```python
from build123d import *

# Parameters (mm, degrees)
SKETCH2_W           = 50
SKETCH2_H           = 60
BOSS_EXTRUDE1_DEPTH = 25
SHELL1_T            = -3
SKETCH3_R           = 11
BOSS_EXTRUDE2_DEPTH = 3
SKETCH4_R           = 4.5
SKETCH4_R_2         = 1
CUT_EXTRUDE1_DEPTH  = 6
CUT_EXTRUDE2_REACH  = 83.24
CUT_EXTRUDE4_REACH  = 83.24
SKETCH7_W           = 4.336684694
SKETCH7_H           = 5
SKETCH7_W_2         = 5
SKETCH7_H_2         = 4.336684694
BOSS_EXTRUDE3_DEPTH = 44
BOSS_EXTRUDE4_REACH = 73.148
SKETCH8_W           = 4
SKETCH8_H           = 3
SKETCH10_W          = 30
SKETCH10_H          = 10
BOSS_EXTRUDE5_DEPTH = 4.5
CUT_EXTRUDE5_START  = -50
SKETCH9_R           = 1.5
CUT_EXTRUDE5_DEPTH  = 50


with BuildPart() as part:
    # Sketch2 → Boss-Extrude1 (new, symmetric)
    with BuildSketch(Plane.XY):
        with Locations((25, -10)):
            Rectangle(SKETCH2_W, SKETCH2_H)
    extrude(amount=BOSS_EXTRUDE1_DEPTH, both=True)

    # Shell1
    shell1_openings = [part.faces().sort_by_distance(p)[0] for p in [
        (25, 20, 0),
        (50, -10, 0),
        (25, -40, 0),
    ]]
    offset(amount=SHELL1_T, openings=shell1_openings, kind=Kind.INTERSECTION)

    # Sketch3 → Boss-Extrude2 (add)
    with BuildSketch(Plane.ZY):
        with Locations(Location((0, 0, 0), (0, 0, 270))):
            Circle(SKETCH3_R)
    extrude(amount=BOSS_EXTRUDE2_DEPTH)

    # Sketch4 → Cut-Extrude1 (cut)
    with BuildSketch(Plane.ZY.offset(3)):
        with Locations(Location((0, 0, 0), (0, 0, 270))):
            Circle(SKETCH4_R)
        with Locations(Location((-8.5, 0, 0), (0, 0, 270))):
            Circle(SKETCH4_R_2)
        with Locations(Location((0, 8.5, 0), (0, 0, 270))):
            Circle(SKETCH4_R_2)
        with Locations(Location((8.5, 0, 0), (0, 0, 270))):
            Circle(SKETCH4_R_2)
        with Locations(Location((0, -8.5, 0), (0, 0, 270))):
            Circle(SKETCH4_R_2)
    extrude(amount=-CUT_EXTRUDE1_DEPTH, mode=Mode.SUBTRACT)

    # Cut-Extrude2: up to this face of the body (flat: up to its plane)
    cut_extrude2_end = Plane(part.part.faces().sort_by_distance((25, -10, -25))[0])
    # Sketch5 → Cut-Extrude2 (cut, up to the picked face)
    with BuildSketch(Plane.XY.offset(25), mode=Mode.PRIVATE) as cut_extrude2_sk1:
        Polygon((0, -24.472587055), (0, -40), (20, -40), align=None)
    cut_extrude2_tool1 = split(extrude(cut_extrude2_sk1.sketch, amount=-CUT_EXTRUDE2_REACH, mode=Mode.PRIVATE), bisect_by=cut_extrude2_end, keep=Keep.BOTH, mode=Mode.PRIVATE)
    # Sketch5 → Cut-Extrude2 (cut, up to the picked face)
    with BuildSketch(Plane.XY.offset(25), mode=Mode.PRIVATE) as cut_extrude2_sk2:
        Polygon((20, 20), (50, -10), (50, 20), align=None)
    cut_extrude2_tool2 = split(extrude(cut_extrude2_sk2.sketch, amount=-CUT_EXTRUDE2_REACH, mode=Mode.PRIVATE), bisect_by=cut_extrude2_end, keep=Keep.BOTH, mode=Mode.PRIVATE)
    add(cut_extrude2_tool1.solids().sort_by(Axis((6.666667, -34.824196, 25), (0, 0, -1)))[0], mode=Mode.SUBTRACT)
    add(cut_extrude2_tool2.solids().sort_by(Axis((40, 10, 25), (0, 0, -1)))[0], mode=Mode.SUBTRACT)

    # Cut-Extrude4: up to this face of the body (flat: up to its plane)
    cut_extrude4_end = Plane(part.part.faces().sort_by_distance((23.370039897, -12.148657051, -25))[0])
    # Sketch6 → Cut-Extrude4 (cut, up to the picked face)
    with BuildSketch(Plane.XY.offset(25), mode=Mode.PRIVATE) as cut_extrude4_sk1:
        Polygon((5, 15), (15.663315306, 15), (45, -14.336684694), (45, -30), (15.272864665, -30), (5, -22.024449411), align=None)
    cut_extrude4_tool1 = split(extrude(cut_extrude4_sk1.sketch, amount=-CUT_EXTRUDE4_REACH, mode=Mode.PRIVATE), bisect_by=cut_extrude4_end, keep=Keep.BOTH, mode=Mode.PRIVATE)
    add(cut_extrude4_tool1.solids().sort_by(Axis((22.200817, -11.008152, 25), (0, 0, -1)))[0], mode=Mode.SUBTRACT)

    # Sketch7 → Boss-Extrude3 (add)
    with BuildSketch(Plane(origin=(0, 0, 22), x_dir=(-1, 0, 0), z_dir=(0, 0, -1))):
        with Locations((-17.831657653, 17.5)):
            Rectangle(SKETCH7_W, SKETCH7_H)
        with Locations((-47.5, -12.168342347)):
            Rectangle(SKETCH7_W_2, SKETCH7_H_2)
        Polygon((-15.272864665, -30), (-20, -30), (-20, -40), (-15.272864665, -36.32999088), align=None)
    extrude(amount=BOSS_EXTRUDE3_DEPTH)

    # Boss-Extrude4: up to this plane
    boss_extrude4_end = Plane(origin=(15.663315306, 15, -85.207972894), z_dir=(0.7071067811865476, 0.7071067811865476, 0))
    # Sketch8 → Boss-Extrude4 (add, up to the surface)
    with BuildSketch(Plane(origin=(-8.788249565, -11.319657172, 0), x_dir=(0.789890553461427, -0.6132478402345992, 0), z_dir=(0.6132478402345992, 0.789890553461427, 0)), mode=Mode.PRIVATE) as boss_extrude4_sk1:
        with Locations((24.294868458, 23.5)):
            Rectangle(SKETCH8_W, SKETCH8_H)
    boss_extrude4_tool1 = split(extrude(boss_extrude4_sk1.sketch, amount=BOSS_EXTRUDE4_REACH, mode=Mode.PRIVATE), bisect_by=boss_extrude4_end, keep=Keep.BOTH, mode=Mode.PRIVATE)
    add(boss_extrude4_tool1.solids().sort_by_distance((10.402038, -26.218433, -23.5))[0])
    # Sketch8 → Boss-Extrude4 (add, up to the surface)
    with BuildSketch(Plane(origin=(-8.788249565, -11.319657172, 0), x_dir=(0.789890553461427, -0.6132478402345992, 0), z_dir=(0.6132478402345992, 0.789890553461427, 0)), mode=Mode.PRIVATE) as boss_extrude4_sk2:
        with Locations((24.294868458, -23.5)):
            Rectangle(SKETCH8_W, SKETCH8_H)
    boss_extrude4_tool2 = split(extrude(boss_extrude4_sk2.sketch, amount=BOSS_EXTRUDE4_REACH, mode=Mode.PRIVATE), bisect_by=boss_extrude4_end, keep=Keep.BOTH, mode=Mode.PRIVATE)
    add(boss_extrude4_tool2.solids().sort_by_distance((10.402038, -26.218433, 23.5))[0])

    # Sketch10 → Boss-Extrude5 (add)
    with BuildSketch(Plane.XY.offset(-22)):
        with Locations((35, -35)):
            Rectangle(SKETCH10_W, SKETCH10_H)
    boss_extrude5 = extrude(amount=BOSS_EXTRUDE5_DEPTH)

    # Mirror1: Boss-Extrude5 across plane
    add(boss_extrude5.mirror(Plane.XY))

    # Sketch9 → Cut-Extrude5 (cut)
    with BuildSketch(Plane.XY.offset(25).offset(CUT_EXTRUDE5_START)):
        with Locations((24.5, -35)):
            Circle(SKETCH9_R)
        with Locations((28.5, -35)):
            Circle(SKETCH9_R)
        with Locations((41.5, -35)):
            Circle(SKETCH9_R)
        with Locations((45.5, -35)):
            Circle(SKETCH9_R)
    extrude(amount=CUT_EXTRUDE5_DEPTH, mode=Mode.SUBTRACT)


solid = part.part
```
Model file for the job. Use its own axes, mm. A direction names the side the tool comes from. Coordinates: 2 decimals unless noted, no trailing zeros. Loops run counter-clockwise (first coordinate to the right, second up) from the corner with the lowest first, then second, coordinate; pieces in that order, holes last. Notation, with made-up numbers: (51, -27.75) - (93, -27.75) arc R25 cw to (93, -1.75) - close; hole circle Ø1 at (-27.75, -18.75). An arc over 180 degrees is marked (long way). Write item = value, one per line. Start each with the question number.
Item 1: Pull direction Z, two halves, no side cores. Call faces 5 (the face through (25, -10, 25)), 6 (the face through (50, -14, 2)), 7 (the face through (-0.042, -4.292, 1.352)), 8 (the face through (25, -6, -22)): +Z half, -Z half, draft (parallel to the pull), parting line (faces both ways), or undercut.
Item 2: Saw through at A-A, the plane z = -21. List the corners of the cut face in (x, y), then the cut area to 3 significant figures.
Item 3: Drop flat-ended pins along their axis: pin 1 Ø2 at (y, z) = (-16, 16) entering from -X; pin 2 Ø5 at (y, z) = (-29, 5) entering from -X; pin 3 Ø3.5 at (x, z) = (10.5, -23) entering from -Y; pin 4 Ø2 at (x, z) = (13, -6) entering from -Y. Give the stop position or say it passes through.
Item 4: Saw through at C-C, the plane y = 16. List the corners of the cut face in (x, z), then the cut area to 3 significant figures.
Item 5: Saw through at B-B, the plane z = 14.5. List the corners of the cut face in (x, y).
Item 6: Saw through at D-D, the plane y = 8.5. List the corners of the cut face in (x, z), then the cut area to 3 significant figures.
Item 7: 3-axis set-ups, long thin cutter, end or side, ignore diameter. For faces 1 (the face through (20, 17, 0)), 2 (the face through (13.65, -28.74, 23.52)), 3 (the face through (45, -12, 0)), 4 (the face through (18, 15, 0)): which of +Z, -Z, +X, -X, +Y, -Y reach the whole face in a straight line?
Item 8: Wall check: probe 1 along X at (y, z) = (-35, 19.5); probe 2 along X at (y, z) = (-12, -18); probe 3 along Z at (x, y) = (2.5, 8.5). Give the ranges that are in metal, low to high. Write a range as [from, to].
Answers:
q1.face_5 = +Z half
q1.face_6 = draft
q1.face_7 = undercut
q1.face_8 = undercut
q2.outline = (0, -24.47) - (3, -26.8) - (3, 20) - (0, 20) - close; (15.27, -36.33) - (20, -40) - (50, -40) - (50, -30) - (15.27, -30) - close; (15.66, 15) - (20, 15) - (20, 20) - (15.66, 20) - close; (45, -14.34) - (50, -14.34) - (50, -10) - (45, -10) - close; hole circle Ø3 at (24.5, -35); hole circle Ø3 at (28.5, -35); hole circle Ø3 at (41.5, -35); hole circle Ø3 at (45.5, -35)
q2.area = 491 mm2
q3.pin_1 = 0
q3.pin_2 = 2.61
q3.pin_3 = -33.98
q3.pin_4 = through
q4.outline = (0, -25) - (24, -25) - (24, -22) - (20, -22) - (20, 22) - (24, 22) - (24, 25) - (0, 25) - close; hole (3, -22) - (15.66, -22) - (15.66, 22) - (3, 22) - close
q4.area = 467 mm2
q5.outline = (0, -24.47) - (3, -26.8) - (3, 20) - (0, 20) - close; (15.27, -36.33) - (20, -40) - (20, -30) - (15.27, -30) - close; (15.66, 15) - (20, 15) - (20, 20) - (15.66, 20) - close; (45, -14.34) - (50, -14.34) - (50, -10) - (45, -10) - close
q6.outline = (-3, -6.98) - (0, -6.98) - (0, -25) - (5, -25) - (5, -22) - (3, -22) - (3, -1) - (-3, -1) - close; (-3, 1) - (3, 1) - (3, 22) - (5, 22) - (5, 25) - (0, 25) - (0, 6.98) - (-3, 6.98) - close; (22.16, -25) - (31.5, -25) - (31.5, -22) - (22.16, -22) - close; (22.16, 22) - (31.5, 22) - (31.5, 25) - (22.16, 25) - close
q6.area = 248 mm2
q7.face_1 = +X, +Y
q7.face_2 = +Z, -Z
q7.face_3 = +Y
q7.face_4 = +X
q8.probe_1 = [15.27, 23], [26, 27], [30, 40], [43, 44], [47, 50]
q8.probe_2 = [0, 3], [45, 50]
q8.probe_3 = [-25, -1], [1, 25]
